from build123d import *

# Parameters (mm, degrees)
SKETCH_R     = 2.25
PAD_DEPTH    = 25
PAD001_DEPTH = 4


with BuildPart() as revolution:
    # Sketch002 → Revolution (revolve)
    with BuildSketch(Plane.XZ):
        Polygon((0, 29.182125), (2.351471, 29.182125), (4.653152, 28.390949), (4.653152, 29.641115), (0, 29.641115), align=None)
    revolve(axis=Axis((0, 0, 0), (0, 0, 1)))


with BuildPart() as tornillo:
    # Sketch → Pad (new body)
    with BuildSketch(Plane.XY):
        Circle(SKETCH_R)
    extrude(amount=PAD_DEPTH)

    # Sketch001 → Pad001 (new body)
    with BuildSketch(Plane.XY.offset(25)):
        Polygon((3.5, 2.020726), (0, 4.041452), (-3.5, 2.020726), (-3.5, -2.020726), (0, -4.041452), (3.5, -2.020726), align=None)
    extrude(amount=PAD001_DEPTH)

    # Cut: cut Revolution
    add(revolution.part, mode=Mode.SUBTRACT)


solid = tornillo.part
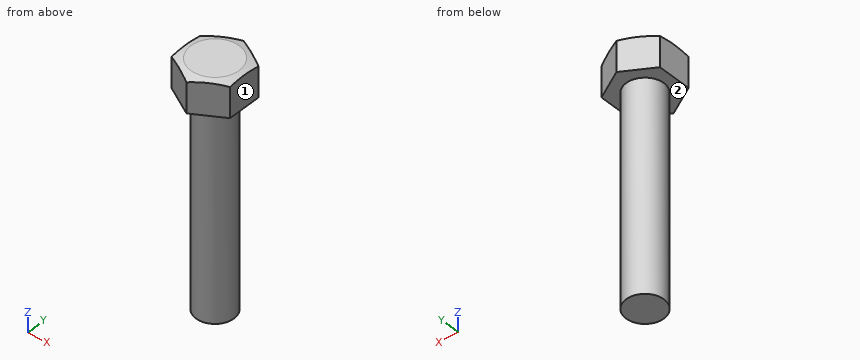
Geometry: final body of the model. Coordinates: model frame, mm. Face numbers are marked on the shaded views. A direction names the side the tool comes from. Coordinates: 2 decimals unless noted, no trailing zeros. Order: outer loops, then holes, each group sorted by start corner. A loop starts at its lowest first (then second) coordinate and runs counter-clockwise, first axis right, second up.
(1) First-contact query: pin 1 (1 mm diameter, centred on y = 1.5, z = 21, fed in from -X); pin 2 (3 mm diameter, centred on x = 1.5, z = 21.5, fed in from -Y); pin 3 (3.5 mm diameter, centred on x = -0.5, y = -1, fed in from -Z); pin 4 (1 mm diameter, centred on y = 0.5, z = 17, fed in from +X). Flat tips, straight axial feed; report the tip coordinate or a pass-through.
(2) Section query C-C (z = 11). Return the cut outline in (x, y), plus the area to 3 significant figures.
(3) Section query A-A (y = 0). Return the cut outline in (x, z), plus the area to 3 significant figures.
(4) Section query B-B (z = 26). Return the cut outline in (x, y).
(5) Material intervals for probe 1 along Z at (x, y) = (-2.5, -0.75); probe 2 along Y at (x, z) = (1, 13); probe 3 along Y at (x, z) = (-2, 19.5), sorted ascending.
(6) Access query for the marked faces 1 and 2. Directions: +Z, -Z, +X, -X, +Y, -Y. A direction counts if a zero-diameter tool reaches every point of the face in a straight line with its end or side. Return the directions, or none.
Solution:
1. pin 1: stops at x = -2.02
1. pin 2: stops at y = -2.25
1. pin 3: stops at z = 0
1. pin 4: stops at x = 2.25
2. outline: circle Ø4.5 at (0, 0)
2. area: 15.9 mm2
3. outline: (-3.5, 25) - (-2.25, 25) - (-2.25, 0) - (2.25, 0) - (2.25, 25) - (3.5, 25) - (3.5, 28.79) - (2.88, 29) - (-2.88, 29) - (-3.5, 28.79) - close
3. area: 140 mm2
4. outline: (-3.5, -2.02) - (0, -4.04) - (3.5, -2.02) - (3.5, 2.02) - (0, 4.04) - (-3.5, 2.02) - close
5. probe 1: z = 25 to 29
5. probe 2: y = -2.02 to 2.02
5. probe 3: y = -1.03 to 1.03
6. face 1: +Z, -Z, +X, +Y, -Y
6. face 2: -Z
